Build history of the part. All positions in model axes, mm. A direction names the side the tool comes from. Round coordinates to 2 decimals unless told otherwise and drop trailing zeros. Order: outer loops, then holes, each group sorted by start corner. A loop starts at its lowest first (then second) coordinate and runs counter-clockwise, first axis right, second up. Notation, with made-up numbers: (-40, 34) -> (-10, 34) arc R28 cw to (-10, 62) -> close; hole circle Ø11 at (80.5, 27). An arc over 180 degrees is marked (long way). Answer as CSV lines item,"result". Start each with the question number.
```python
from build123d import *

# Parameters (mm, degrees)
SKETCH1_W           = 4
SKETCH1_H           = 120
BOSS_EXTRUDE1_DEPTH = 100
BOSS_EXTRUDE2_DEPTH = 10
BOSS_EXTRUDE3_DEPTH = 100


with BuildPart() as part:
    # Sketch1 → Boss-Extrude1 (new body)
    with BuildSketch(Plane.XY):
        with Locations((2, 60)):
            Rectangle(SKETCH1_W, SKETCH1_H)
    extrude(amount=BOSS_EXTRUDE1_DEPTH)

    # Sketch2 → Boss-Extrude2 (add)
    with BuildSketch(Plane(origin=(4, 0, 0), x_dir=(0, 0, -1), z_dir=(1, 0, 0))):
        Polygon((-100, 0), (-100, 1), (0, 9.748866353), (0, 0), align=None)
    extrude(amount=BOSS_EXTRUDE2_DEPTH)

    # Sketch4 → Boss-Extrude3 (add)
    with BuildSketch(Plane(origin=(0, 0, 0), x_dir=(-1, 0, 0), z_dir=(0, 0, -1))):
        Polygon((-14, 0), (-14, 49.748866353), (-71.74011537, 107.488981723), (-74.568542495, 104.660554598), (-18, 48.092012103), (-18, 0), align=None)
    extrude(amount=-BOSS_EXTRUDE3_DEPTH)


solid = part.part
```
Q1. Slice it at A-A, the plane y = 28. Write the cut outline in (x, z), plus the area to 3 significant figures.
Q2. Probe L1, parallel to X at y = 21.5, z = 70; L2, parallel to X at y = 107, z = 52.5; L3, parallel to Y at x = 60.5, z = 30.5. List the from-to ranges inside material, lowest first.
Q3. Flat gauge pins, fed straight in: pin 1 Ø6 at (y, z) = (65.5, 28.5) entering from +X; pin 2 Ø10 at (x, z) = (58.5, 74) entering from -Y; pin 3 Ø14.5 at (y, z) = (31, 35.5) entering from +X; pin 4 Ø1 at (x, y) = (36, 63) entering from -Z. Where does each tip first touch, or does it go through?
Q4. Slice it at D-D, the plane y = 92. Write the cut outline in (x, z).
Q5. Slice it at B-B, the plane z = 33. Write the cut outline in (x, y).
Q6. Slice it at C-C, the plane x = 12.5. Write the cut outline in (y, z), plus the area to 3 significant figures.
Q7. Two-plate mould, pull along X, no slides. Class faces 1 (the face through (4, 60, 49)), 2 (the face through (0, 59, 49)), 3 (the face through (2, 120, 49)): +X half, -X half, draft (parallel to the pull), parting line (faces both ways), or undercut.
Q8. Which spindle directions (+Z, -Z, +X, -X, +Y, -Y) get a long thin tool onto all of the face, cutting with end or side? Do faces 4 (the face through (8.93, 5.313, 50.7)), 5 (the face through (18, 24, 49)), 6 (the face through (42.466, 78.215, 49.3)). Say none if no direction does.
Solutions:
1,outline,"(0, 0) -> (4, 0) -> (4, 100) -> (0, 100) -> close; (14, 0) -> (18, 0) -> (18, 100) -> (14, 100) -> close"
1,area,"800 mm2"
2,L1,"x = 0 to 4, 14 to 18"
2,L2,"x = 0 to 4, 71.25 to 72.23"
2,L3,"y = 90.59 to 96.25"
3,pin 1,"stops at x = 38.41"
3,pin 2,"stops at y = 83.59"
3,pin 3,"stops at x = 18"
3,pin 4,"passes through"
4,outline,"(0, 0) -> (4, 0) -> (4, 100) -> (0, 100) -> close; (56.25, 0) -> (61.91, 0) -> (61.91, 100) -> (56.25, 100) -> close"
5,outline,"(0, 0) -> (18, 0) -> (18, 48.09) -> (74.57, 104.66) -> (71.74, 107.49) -> (14, 49.75) -> (14, 6.86) -> (4, 6.86) -> (4, 120) -> (0, 120) -> close"
6,outline,"(0, 0) -> (9.75, 0) -> (1, 100) -> (0, 100) -> close"
6,area,"537 mm2"
7,face 1,"undercut"
7,face 2,"-X half"
7,face 3,"draft"
8,face 4,"+Z, +Y"
8,face 5,"+Z, -Z, +X, -Y"
8,face 6,"+Z, -Z, +Y"
